Can you work these out from the drawing? Everything is in mm from the part's minimum corner. A direction names the side the tool comes from. Coordinates: 2 decimals unless noted, no trailing zeros. Loops run counter-clockwise (first coordinate to the right, second up) from the corner with the lowest first, then second, coordinate; pieces in that order, holes last. Notation, with made-up numbers: (-1.75, 85) - (19.25, 85) arc R9 cw to (19.25, 95) - close; hole circle Ø7 at (1.25, 40). An arc over 180 degrees is marked (long way). Use CSV: the item, a comma, the result in double quotes.
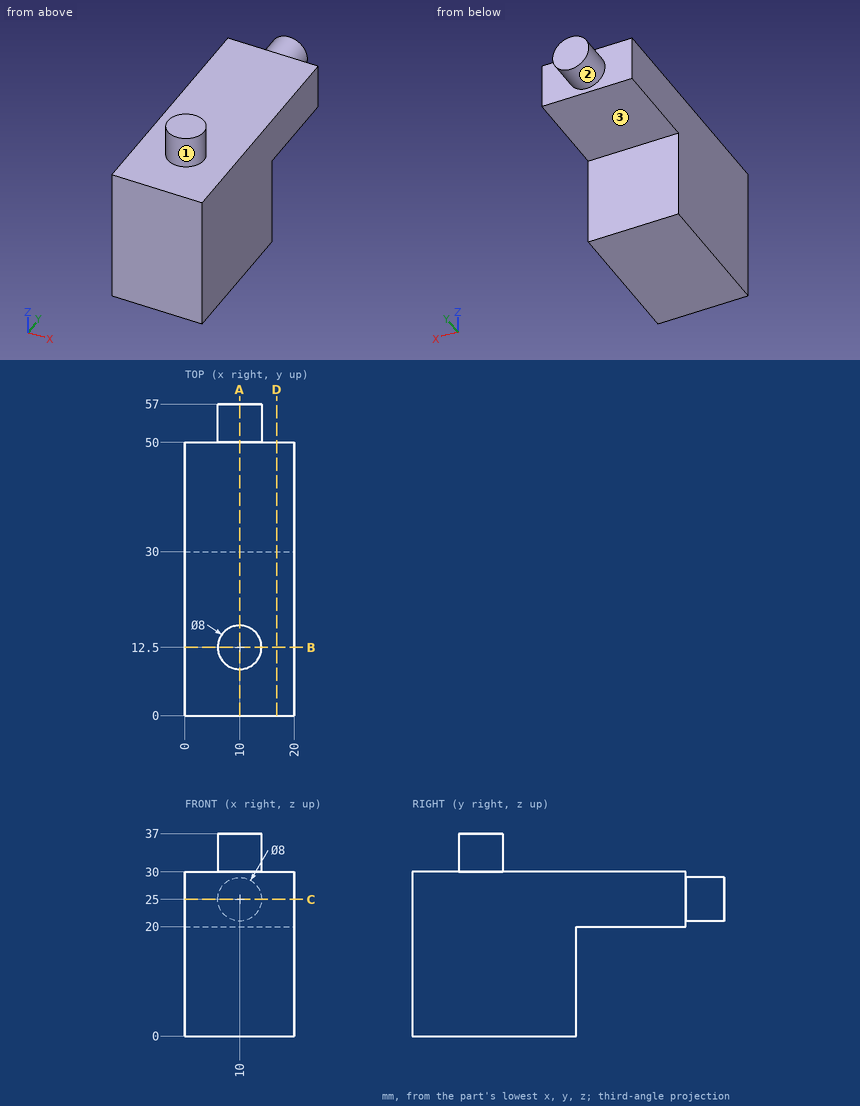
(1) Suppose I cut it at A-A (x = 10). Write out the boundary of the cut face in (y, z), plus the area to 3 significant figures.
Computed:
outline,"(0, 0) - (30, 0) - (30, 20) - (50, 20) - (50, 21) - (57, 21) - (57, 29) - (50, 29) - (50, 30) - (16.5, 30) - (16.5, 37) - (8.5, 37) - (8.5, 30) - (0, 30) - close"
area,"1,210 mm²"
(2) Suppose I cut it at C-C (z = 25). Write out the boundary of the cut face in (x, y), plus the area to 3 significant figures.
Computed:
outline,"(0, 0) - (20, 0) - (20, 50) - (14, 50) - (14, 57) - (6, 57) - (6, 50) - (0, 50) - close"
area,"1,060 mm²"
(3) Please list where these lines run through material, in increasing order: line 1 (Z direction, x = 2.25, y = 22); line 2 (Z direction, x = 18.25, y = 35).
Computed:
line 1,"z = 0 to 30"
line 2,"z = 20 to 30"
(4) Which directions (+Z, -Z, +X, -X, +Y, -Y) give clear straight access to the entire face, cutting with the end or side of a thin tool? Please do the marked faces 1, 2 and 3.
Computed:
face 1,"+Z"
face 2,"+Y"
face 3,"-Z, +X, -X, +Y"
(5) Suppose I cut it at D-D (x = 16.75). Write out the boundary of the cut face in (y, z).
Computed:
outline,"(0, 0) - (30, 0) - (30, 20) - (50, 20) - (50, 30) - (0, 30) - close"
(6) Will these pins go through, and if not, where does the flat tip stop? pin 1 (6 mm diameter, centred on x = 11, y = 34, fed in from +Z); pin 2 (6 mm diameter, centred on x = 7, z = 8, fed in from +Y); pin 3 (3 mm diameter, centred on x = 7.5, y = 43.5, fed in from -Z).
Computed:
pin 1,"stops at z = 30"
pin 2,"stops at y = 30"
pin 3,"stops at z = 20"
(7) Suppose I cut it at B-B (y = 12.5). Write out the boundary of the cut face in (x, z).
Computed:
outline,"(0, 0) - (20, 0) - (20, 30) - (14, 30) - (14, 37) - (6, 37) - (6, 30) - (0, 30) - close"
